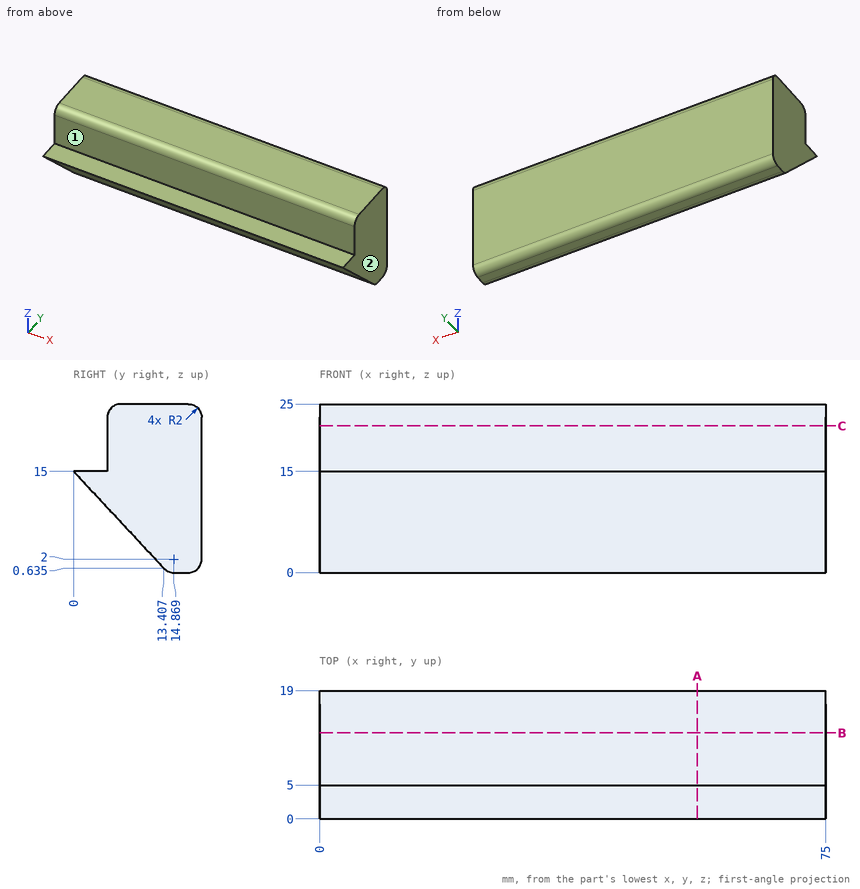
Study the drawing (mm; zero at the part's minimum x, y, z) and answer. A direction names the side the tool comes from. Give positions to 0.01 mm unless a question says otherwise; leave off trailing zeros. Write each loop counter-clockwise with the first axis right and the second up, starting at its lowest first coordinate (ties: lowest second). Pieces come first, ordered by that corner, then holes. Notation, with made-up numbers: (43.25, 64.25) - (83.25, 64.25) arc R20 ccw to (83.25, 75.25) - close; hole circle Ø11 at (72, -30). An arc over 180 degrees is marked (long way). Use a Markdown table: item, result.
1. Each of these flat-tipped pins is pushed along its axis until it touches: P1, Ø4, axis at x = 32.5, y = 7, coming from the -Z side; P2, Ø2.5, axis at x = 22.5, y = 1.5, coming from the +Z side; P3, Ø6, axis at x = 46, z = 11, coming from the -Y side. Where does it stop, or does it pass through?
Values follow:
| item | result |
|---|---|
| P1 | stops at z = 5.36 |
| P2 | stops at z = 15 |
| P3 | stops at y = 0.93 |
2. Section C-C on z = 21.75 is taken. Write down the section's boundary in (x, y).
Values follow:
| item | result |
|---|---|
| outline | (0, 5) - (75, 5) - (75, 19) - (0, 19) - close |
3. A tool of negligible diameter and unlimited length cuts with its end or side. For the marked faces 1 and 2, from which of +Z, -Z, +X, -X, +Y, -Y can it reach the whole face along a straight path? Write none if from no direction.
Values follow:
| item | result |
|---|---|
| face 1 | +Z, +X, -X, -Y |
| face 2 | +Z, -Z, +X, +Y, -Y |
4. Find the intervals of material crossed by probe 1 along Z at (x, y) = (26.5, 14.75); probe 2 along Y at (x, z) = (62, 18); probe 3 along Y at (x, z) = (50, 5) (1 decimal), in increasing order. Write a range as from..to.
Values follow:
| item | result |
|---|---|
| probe 1 | z = 0..25 |
| probe 2 | y = 5..19 |
| probe 3 | y = 9.3..19 |
5. Section A-A on x = 56 is taken. Write down the section's boundary in (y, z) (1 decimal), plus the area to 3 significant figures.
Values follow:
| item | result |
|---|---|
| outline | (0, 15) - (13.4, 0.6) arc R2 ccw to (14.9, 0) - (17, 0) arc R2 ccw to (19, 2) - (19, 23) arc R2 ccw to (17, 25) - (7, 25) arc R2 ccw to (5, 23) - (5, 15) - close |
| area | 317 mm² |
6. Section B-B on y = 12.75 is taken. Write down the section's boundary in (x, z).
Values follow:
| item | result |
|---|---|
| outline | (0, 1.34) - (75, 1.34) - (75, 25) - (0, 25) - close |
